Answer from the drawing. Dimensions are ordinates in mm from the lowest x, y and z of the part. Give positions to 0.01 mm unless a question says otherwise; leave off trailing zeros. Loops run counter-clockwise (first coordinate to the right, second up) from the corner with the lowest first, then second, coordinate; pieces in that order, holes last. Notation, with made-up numbers: (25, 34) - (72, 34) arc R17 ccw to (72, 66) - close; hole circle Ø3 at (-6, 53). An arc over 180 degrees is marked (long way). One line per item, written item: value.
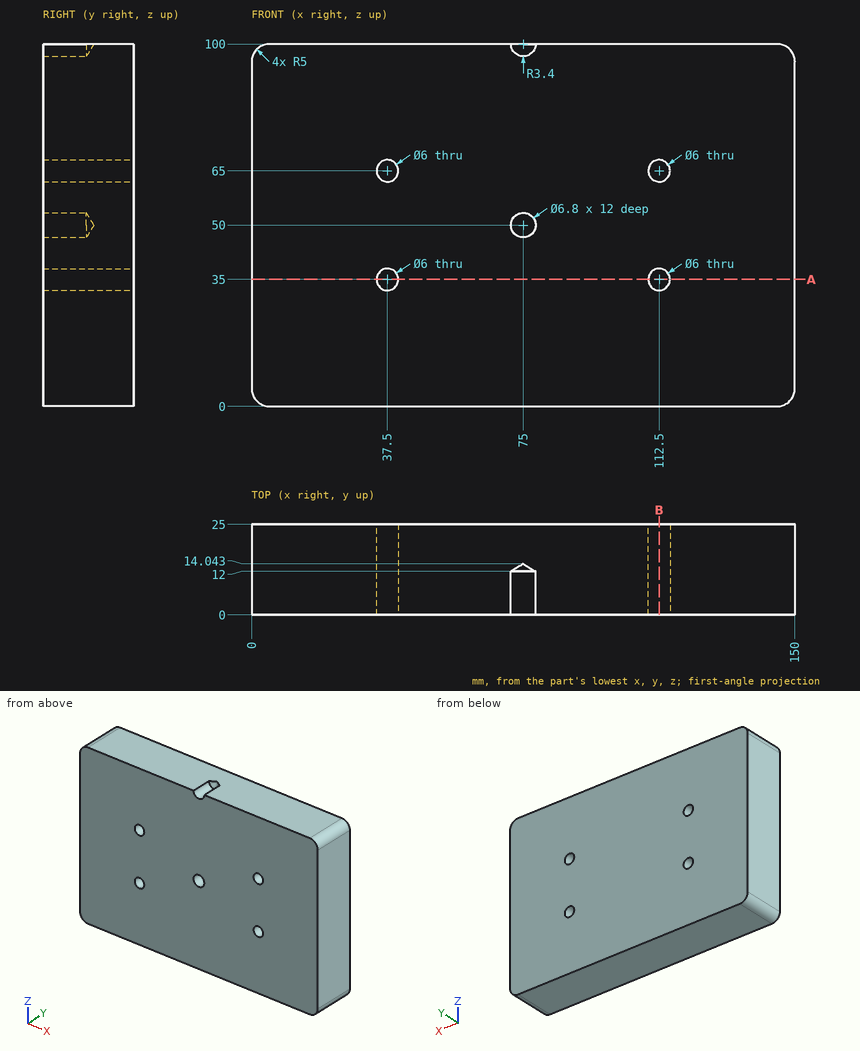
1. Section B-B (x = 112.5) is taken. Write down the section's boundary in (y, z), and give its area (3 significant figures).
Output:
outline: (0, 0) - (25, 0) - (25, 32) - (0, 32) - close; (0, 38) - (25, 38) - (25, 62) - (0, 62) - close; (0, 68) - (25, 68) - (25, 100) - (0, 100) - close
area: 2,200 mm²
2. Section A-A (z = 35) is taken. Write down the section's boundary in (x, y).
Output:
outline: (0, 0) - (34.5, 0) - (34.5, 25) - (0, 25) - close; (40.5, 0) - (109.5, 0) - (109.5, 25) - (40.5, 25) - close; (115.5, 0) - (150, 0) - (150, 25) - (115.5, 25) - close
3. Find the intervals of material crossed by line 1 along Z through (x, y) = (37.5, 17.75); line 2 along X through (y, z) = (4.25, 50), in increasing order.
Output:
line 1: z = 0 to 32, 38 to 62, 68 to 100
line 2: x = 0 to 71.6, 78.4 to 150
4. A flat-ended cylindrical pin translates along its axis: pin 1 Ø3.5 at (x, z) = (37.5, 65) entering from -Y. Find the tip coordinate at first contact, or state that the pin passes through.
Output:
pin 1: passes through
